The model under review builds one solid part; all positions refer to its coordinate system, in mm. Give positions to 0.01 mm unless a question says otherwise; leave off trailing zeros. Loops run counter-clockwise (first coordinate to the right, second up) from the corner with the lowest first, then second, coordinate; pieces in that order, holes last. Notation, with made-up numbers: (11.5, 81) - (28.5, 81) arc R12 cw to (28.5, 85) - close; hole circle Ø7 at (61, 19). An arc over 180 degrees is marked (long way). Return JSON: item names as keys, results as strings. Group by question number.
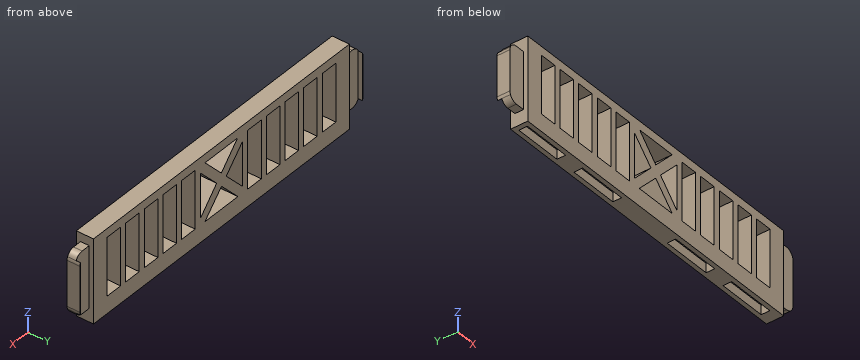
from build123d import *

# Parameters (mm, degrees)
F0_W     = 8
F0_H     = 26.900017
F1_DEPTH = 6
F2_DEPTH = 2
F3_DEPTH = 8
F4_W     = 23
F4_H     = 4
F4_W_2   = 22.5
F5_DEPTH = 5


with BuildPart() as f1:
    # F0 (on Front) → F1 (new body)
    with BuildSketch(Plane.XZ):
        with BuildLine():
            Line((-85.422808, 9.222019), (-85.422808, 31.025267))
            ThreePointArc((-85.422808, 31.025267), (-85.64706, 30.296735), (-85.722808, 29.538243))
            Line((-85.722808, 29.538243), (-85.722808, 10.709043))
            ThreePointArc((-85.722808, 10.709043), (-85.64706, 9.950551), (-85.422808, 9.222019))
        make_face()
        with BuildLine():
            ThreePointArc((81.277192, 31.73826), (81.201444, 32.496752), (80.977192, 33.225284))
            Line((80.977192, 33.225284), (80.977192, 9.222019))
            ThreePointArc((80.977192, 9.222019), (81.201444, 9.950551), (81.277192, 10.709043))
            Line((81.277192, 10.709043), (81.277192, 31.73826))
        make_face()
        with BuildLine():
            Line((77.441792, 35.57366), (73.277192, 35.57366))
            Line((73.277192, 35.57366), (73.277192, 11.555429))
            Line((73.277192, 11.555429), (73.277192, 8.673643))
            Line((73.277192, 8.673643), (73.277192, 6.873643))
            Line((73.277192, 6.873643), (77.441792, 6.873643))
            ThreePointArc((77.441792, 6.873643), (79.563932, 7.514232), (80.977192, 9.222019))
            Line((80.977192, 9.222019), (80.977192, 33.225284))
            ThreePointArc((80.977192, 33.225284), (79.563932, 34.93307), (77.441792, 35.57366))
        make_face()
        Polygon((-69.722808, 39.57366), (-77.722808, 39.57366), (-77.722808, 35.57366), (-77.722808, 33.373643), (-77.722808, 15.555412), (-77.722808, 8.673643), (-77.722808, 6.873643), (-77.722808, 0.673643), (-69.722808, 0.673643), (65.277192, 0.673643), (73.277192, 0.673643), (73.277192, 6.873643), (73.277192, 8.673643), (73.277192, 11.555429), (73.277192, 35.57366), (73.277192, 39.57366), (65.277192, 39.57366), align=None)
        Polygon((-11.958453, 8.673643), (-2.267612, 19.087933), (7.512836, 8.673643), align=None, mode=Mode.SUBTRACT)
        with Locations((-65.722808, 22.123651)):
            Rectangle(F0_W, F0_H, mode=Mode.SUBTRACT)
        with Locations((-54.722808, 22.123651)):
            Rectangle(F0_W, F0_H, mode=Mode.SUBTRACT)
        with Locations((-43.722808, 22.123651)):
            Rectangle(F0_W, F0_H, mode=Mode.SUBTRACT)
        with Locations((-32.722808, 22.123651)):
            Rectangle(F0_W, F0_H, mode=Mode.SUBTRACT)
        with Locations((-21.722808, 22.123651)):
            Rectangle(F0_W, F0_H, mode=Mode.SUBTRACT)
        Polygon((-14.722808, 11.648091), (-14.722808, 32.350313), (-5.058615, 22.059812), align=None, mode=Mode.SUBTRACT)
        Polygon((0.600276, 22.169918), (10.277192, 32.569243), (10.277192, 11.648091), align=None, mode=Mode.SUBTRACT)
        with Locations((17.277192, 22.123651)):
            Rectangle(F0_W, F0_H, mode=Mode.SUBTRACT)
        with Locations((28.277192, 22.123651)):
            Rectangle(F0_W, F0_H, mode=Mode.SUBTRACT)
        with Locations((39.277192, 22.123651)):
            Rectangle(F0_W, F0_H, mode=Mode.SUBTRACT)
        with Locations((50.277192, 22.123651)):
            Rectangle(F0_W, F0_H, mode=Mode.SUBTRACT)
        with Locations((61.277192, 22.123651)):
            Rectangle(F0_W, F0_H, mode=Mode.SUBTRACT)
        Polygon((7.484984, 35.57366), (-2.165283, 25.176943), (-11.727135, 35.57366), align=None, mode=Mode.SUBTRACT)
        with BuildLine():
            Line((-77.722808, 15.555412), (-77.722808, 33.373643))
            Line((-77.722808, 33.373643), (-81.887408, 33.373643))
            ThreePointArc((-81.887408, 33.373643), (-84.009549, 32.733053), (-85.422808, 31.025267))
            Line((-85.422808, 31.025267), (-85.422808, 9.222019))
            ThreePointArc((-85.422808, 9.222019), (-84.009549, 7.514232), (-81.887408, 6.873643))
            Line((-81.887408, 6.873643), (-77.722808, 6.873643))
            Line((-77.722808, 6.873643), (-77.722808, 8.673643))
            Line((-77.722808, 8.673643), (-77.722808, 15.555412))
        make_face()
    extrude(amount=F1_DEPTH)

    # F0 (on Front) → F2 (cut)
    with BuildSketch(Plane.XZ):
        with BuildLine():
            Line((-77.722808, 15.555412), (-77.722808, 33.373643))
            Line((-77.722808, 33.373643), (-81.887408, 33.373643))
            ThreePointArc((-81.887408, 33.373643), (-84.009549, 32.733053), (-85.422808, 31.025267))
            Line((-85.422808, 31.025267), (-85.422808, 9.222019))
            ThreePointArc((-85.422808, 9.222019), (-84.009549, 7.514232), (-81.887408, 6.873643))
            Line((-81.887408, 6.873643), (-77.722808, 6.873643))
            Line((-77.722808, 6.873643), (-77.722808, 8.673643))
            Line((-77.722808, 8.673643), (-77.722808, 15.555412))
        make_face()
        with BuildLine():
            Line((77.441792, 35.57366), (73.277192, 35.57366))
            Line((73.277192, 35.57366), (73.277192, 11.555429))
            Line((73.277192, 11.555429), (73.277192, 8.673643))
            Line((73.277192, 8.673643), (73.277192, 6.873643))
            Line((73.277192, 6.873643), (77.441792, 6.873643))
            ThreePointArc((77.441792, 6.873643), (79.563932, 7.514232), (80.977192, 9.222019))
            Line((80.977192, 9.222019), (80.977192, 33.225284))
            ThreePointArc((80.977192, 33.225284), (79.563932, 34.93307), (77.441792, 35.57366))
        make_face()
    extrude(amount=F2_DEPTH, mode=Mode.SUBTRACT)

    # F0 (on Front) → F3 (join)
    with BuildSketch(Plane.XZ):
        Polygon((-69.722808, 39.57366), (-77.722808, 39.57366), (-77.722808, 35.57366), (-77.722808, 33.373643), (-77.722808, 15.555412), (-77.722808, 8.673643), (-77.722808, 6.873643), (-77.722808, 0.673643), (-69.722808, 0.673643), (65.277192, 0.673643), (73.277192, 0.673643), (73.277192, 6.873643), (73.277192, 8.673643), (73.277192, 11.555429), (73.277192, 35.57366), (73.277192, 39.57366), (65.277192, 39.57366), align=None)
        Polygon((-11.958453, 8.673643), (-2.267612, 19.087933), (7.512836, 8.673643), align=None, mode=Mode.SUBTRACT)
        with Locations((-65.722808, 22.123651)):
            Rectangle(F0_W, F0_H, mode=Mode.SUBTRACT)
        with Locations((-54.722808, 22.123651)):
            Rectangle(F0_W, F0_H, mode=Mode.SUBTRACT)
        with Locations((-43.722808, 22.123651)):
            Rectangle(F0_W, F0_H, mode=Mode.SUBTRACT)
        with Locations((-32.722808, 22.123651)):
            Rectangle(F0_W, F0_H, mode=Mode.SUBTRACT)
        with Locations((-21.722808, 22.123651)):
            Rectangle(F0_W, F0_H, mode=Mode.SUBTRACT)
        Polygon((-14.722808, 11.648091), (-14.722808, 32.350313), (-5.058615, 22.059812), align=None, mode=Mode.SUBTRACT)
        Polygon((0.600276, 22.169918), (10.277192, 32.569243), (10.277192, 11.648091), align=None, mode=Mode.SUBTRACT)
        with Locations((17.277192, 22.123651)):
            Rectangle(F0_W, F0_H, mode=Mode.SUBTRACT)
        with Locations((28.277192, 22.123651)):
            Rectangle(F0_W, F0_H, mode=Mode.SUBTRACT)
        with Locations((39.277192, 22.123651)):
            Rectangle(F0_W, F0_H, mode=Mode.SUBTRACT)
        with Locations((50.277192, 22.123651)):
            Rectangle(F0_W, F0_H, mode=Mode.SUBTRACT)
        with Locations((61.277192, 22.123651)):
            Rectangle(F0_W, F0_H, mode=Mode.SUBTRACT)
        Polygon((7.484984, 35.57366), (-2.165283, 25.176943), (-11.727135, 35.57366), align=None, mode=Mode.SUBTRACT)
    extrude(amount=F3_DEPTH)

    # F4 (on Top) → F5 (cut)
    with BuildSketch(Plane.XY):
        Polygon((-75.366058, -1.990048), (-75.366058, -5.990048), (-52.866058, -5.990048), (-52.866058, -3.990048), (-52.866058, -1.990048), align=None)
        Polygon((-42.866058, -1.990048), (-42.866058, -5.990048), (-19.866058, -5.990048), (-19.866058, -3.990048), (-19.866058, -1.990048), align=None)
        with Locations((23.633942, -3.990048)):
            Rectangle(F4_W, F4_H)
        with Locations((56.383942, -3.990048)):
            Rectangle(F4_W_2, F4_H)
    extrude(amount=F5_DEPTH, mode=Mode.SUBTRACT)


solid = f1.part
Item 1: For L1, parallel to Z at x = 30.5, y = -1.75; L2, parallel to Z at x = -9, y = -1; L3, parallel to Y at x = -74, z = 4, list the stretches that pass through material, from the lowest coordinate up. Write a range as from..to.
Item 2: Take a section at B-B (x = -57). State the section outline as (y, z) points.
Item 3: Take a section at A-A (x = 38). State the section outline as (y, z) points, then the cut area to 3 significant figures.
Item 4: For P1, Ø3, axis at x = 62.5, y = -4, coming from the -Z side; P2, Ø2, axis at y = -3, z = 3.5, coming from the -X side; P3, Ø4, axis at x = 52, y = -3.5, coming from the -Z side; P4, Ø2.5, axis at x = 77, z = 23.5, coming from the -Y side, all flat-tipped, find the tip position at first contact; note any pin that passes through.
Item 5: Take a section at C-C (y = -4.5). State how many separate pieces and enclosed holes the cut face has, then the cut area to 3 significant figures.
Check sheet entries:
{
 "1": {"L1": "z = 0.67..8.67, 35.57..39.57", "L2": "z = 0.67..8.67, 11.85..17.81, 26.26..32.61, 35.57..39.57", "L3": "y = -8..-5.99, -1.99..0"},
 "2": {"outline": "(-8, 0.67) - (-5.99, 0.67) - (-5.99, 5) - (-1.99, 5) - (-1.99, 0.67) - (0, 0.67) - (0, 8.67) - (-8, 8.67) - close; (-8, 35.57) - (0, 35.57) - (0, 39.57) - (-8, 39.57) - close"},
 "3": {"outline": "(-8, 0.67) - (0, 0.67) - (0, 8.67) - (-8, 8.67) - close; (-8, 35.57) - (0, 35.57) - (0, 39.57) - (-8, 39.57) - close", "area": "96.0 mm^2"},
 "4": {"P1": "stops at z = 5", "P2": "stops at x = -77.72", "P3": "stops at z = 0.67", "P4": "stops at y = -6"},
 "5": {"separate pieces": "1", "enclosed holes": "14", "area": "3,350 mm^2"}
}
